For this review, take the finished solid that the model builds, in its own axes (mm). Face numbers are marked on the shaded views. A direction names the side the tool comes from. Coordinates: 2 decimals unless noted, no trailing zeros. Order: outer loops, then holes, each group sorted by start corner. A loop starts at its lowest first (then second) coordinate and runs counter-clockwise, first axis right, second up.
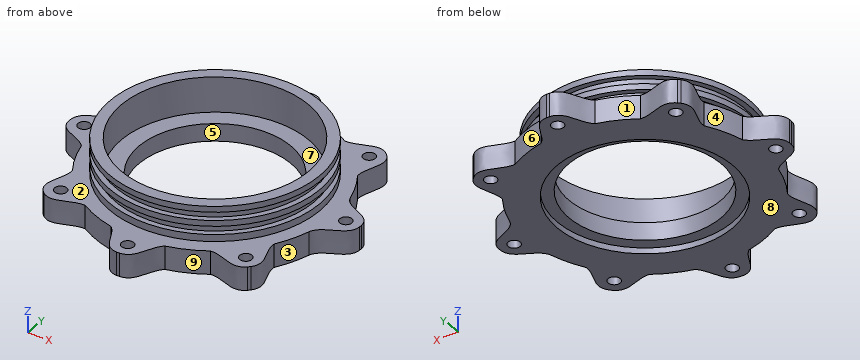
from build123d import *

# Parameters (mm, degrees)
SKETCH1_R           = 44.85
BOSS_EXTRUDE1_DEPTH = 15
SKETCH2_R           = 62.5
BOSS_EXTRUDE2_DEPTH = 10
SKETCH3_R           = 40
CUT_EXTRUDE1_DEPTH  = 15
SKETCH4_W           = 3.5
SKETCH4_H           = 3.724799257
SKETCH7_R           = 2.6
CUT_EXTRUDE4_DEPTH  = 92.855865354
CIRPATTERN1_COUNT   = 8
SKETCH9_R           = 37.5
CUT_EXTRUDE6_DEPTH  = 2.5
SKETCH10_R          = 32.5
CUT_EXTRUDE7_DEPTH  = 92.207181735
CUT_EXTRUDE12_DEPTH = 10


with BuildPart() as part:
    # Sketch1 → Boss-Extrude1 (new body)
    with BuildSketch(Plane.XY):
        Circle(SKETCH1_R)
    extrude(amount=BOSS_EXTRUDE1_DEPTH)

    # Sketch2 → Boss-Extrude2 (add)
    with BuildSketch(Plane(origin=(0, 0, 0), x_dir=(-1, 0, 0), z_dir=(0, 0, -1))):
        Circle(SKETCH2_R)
    extrude(amount=BOSS_EXTRUDE2_DEPTH)

    # Sketch3 → Cut-Extrude1 (cut)
    with BuildSketch(Plane.XY.offset(15)):
        Circle(SKETCH3_R)
    extrude(amount=-CUT_EXTRUDE1_DEPTH, mode=Mode.SUBTRACT)

    # Sketch4 → Cut-Revolve1 (revolve, cut)
    with BuildSketch(Plane(origin=(0, 0, 0), x_dir=(0, 0, -1), z_dir=(1, 0, 0))):
        with Locations((-4.75, 44.412399629)):
            Rectangle(SKETCH4_W, SKETCH4_H)
        with Locations((-10.75, 44.412399629)):
            Rectangle(SKETCH4_W, SKETCH4_H)
    revolve(axis=Axis((0, 0, -42.713110189), (0, 0, 1)), mode=Mode.SUBTRACT)

    # Sketch7 → Cut-Extrude4 (cut, through all)
    with BuildSketch(Plane(origin=(0, 0, -10), x_dir=(-1, 0, 0), z_dir=(0, 0, -1))):
        with Locations((56.25, 0)):
            Circle(SKETCH7_R)
    cut_extrude4 = extrude(amount=-CUT_EXTRUDE4_DEPTH, mode=Mode.SUBTRACT)

    # CirPattern1: Cut-Extrude4 ×8 about axis
    cirpattern1_axis = Axis((0, 0, 0), (0, 0, 1))
    for i in range(1, CIRPATTERN1_COUNT):
        add(cut_extrude4.rotate(cirpattern1_axis, i * 360 / CIRPATTERN1_COUNT), mode=Mode.SUBTRACT)

    # Sketch9 → Cut-Extrude6 (cut)
    with BuildSketch(Plane(origin=(0, 0, -10), x_dir=(-1, 0, 0), z_dir=(0, 0, -1))):
        Circle(SKETCH9_R)
    extrude(amount=-CUT_EXTRUDE6_DEPTH, mode=Mode.SUBTRACT)

    # Sketch10 → Cut-Extrude7 (cut, through all)
    with BuildSketch(Plane(origin=(0, 0, -7.5), x_dir=(-1, 0, 0), z_dir=(0, 0, -1))):
        Circle(SKETCH10_R)
    extrude(amount=-CUT_EXTRUDE7_DEPTH, mode=Mode.SUBTRACT)

    # Sketch16 → Cut-Extrude12 (cut)
    with BuildSketch(Plane.XY):
        with BuildLine():
            ThreePointArc((43.328890761, 26.899948428), (46.799594325, 20.268151644), (49.262217141, 13.1997713))
            add(Edge.make_bspline(
                [(62.49659969, 0.651941114), (62.158853916, 8.013585107), (51.562803867, 6.904158473), (49.262217141, 13.1997713)],
                knots=[0.027770853, 0.027770853, 0.027770853, 0.027770853, 1, 1, 1, 1], degree=3))
            ThreePointArc((62.49659969, 0.651941114), (57.723829207, 23.962669753), (44.584603378, 43.800264173))
            add(Edge.make_bspline(
                [(44.584603378, 43.800264173), (49.25969449, 38.753062003), (42.704327463, 32.585285285), (43.328890761, 26.899948428)],
                knots=[0.023286113, 0.023286113, 0.023286113, 0.023286113, 0.913122258, 0.913122258, 0.913122258, 0.913122258], degree=3))
        make_face()
        with BuildLine():
            add(Edge.make_bspline(
                [(62.49659969, -0.651941114), (62.158853916, -8.013585107), (51.562803867, -6.904158473), (49.262217141, -13.1997713)],
                knots=[0.027770853, 0.027770853, 0.027770853, 0.027770853, 1, 1, 1, 1], degree=3))
            ThreePointArc((49.262217141, -13.1997713), (46.799594325, -20.268151644), (43.328890761, -26.899948428))
            add(Edge.make_bspline(
                [(44.584603378, -43.800264173), (49.25969449, -38.753062003), (42.704327463, -32.585285285), (43.328890761, -26.899948428)],
                knots=[0.023286113, 0.023286113, 0.023286113, 0.023286113, 0.913122258, 0.913122258, 0.913122258, 0.913122258], degree=3))
            ThreePointArc((44.584603378, -43.800264173), (57.723829207, -23.962669753), (62.49659969, -0.651941114))
        make_face()
        with BuildLine():
            ThreePointArc((11.617016531, 49.659288425), (19.516855051, 47.117856158), (26.899948428, 43.328890761))
            add(Edge.make_bspline(
                [(43.800264173, 44.584603378), (38.753062003, 49.25969449), (32.585285285, 42.704327463), (26.899948428, 43.328890761)],
                knots=[0.023286113, 0.023286113, 0.023286113, 0.023286113, 0.913122258, 0.913122258, 0.913122258, 0.913122258], degree=3))
            ThreePointArc((43.800264173, 44.584603378), (23.917714523, 57.742470782), (0.55461157, 62.4975392))
            add(Edge.make_bspline(
                [(0.55461157, 62.4975392), (7.429311079, 62.234416947), (7.155243343, 53.237795727), (11.617016531, 49.659288425)],
                knots=[0.023286113, 0.023286113, 0.023286113, 0.023286113, 0.913122258, 0.913122258, 0.913122258, 0.913122258], degree=3))
        make_face()
        with BuildLine():
            add(Edge.make_bspline(
                [(43.800264173, -44.584603378), (38.753062003, -49.25969449), (32.585285285, -42.704327463), (26.899948428, -43.328890761)],
                knots=[0.023286113, 0.023286113, 0.023286113, 0.023286113, 0.913122258, 0.913122258, 0.913122258, 0.913122258], degree=3))
            ThreePointArc((26.899948428, -43.328890761), (19.516855051, -47.117856158), (11.617016531, -49.659288425))
            add(Edge.make_bspline(
                [(0.55461157, -62.4975392), (7.429311079, -62.234416947), (7.155243343, -53.237795727), (11.617016531, -49.659288425)],
                knots=[0.023286113, 0.023286113, 0.023286113, 0.023286113, 0.913122258, 0.913122258, 0.913122258, 0.913122258], degree=3))
            ThreePointArc((0.55461157, -62.4975392), (23.917714523, -57.742470782), (43.800264173, -44.584603378))
        make_face()
        with BuildLine():
            ThreePointArc((-26.899948428, 43.328890761), (-19.516855051, 47.117856158), (-11.617016531, 49.659288425))
            add(Edge.make_bspline(
                [(-0.55461157, 62.4975392), (-7.429311079, 62.234416947), (-7.155243343, 53.237795727), (-11.617016531, 49.659288425)],
                knots=[0.023286113, 0.023286113, 0.023286113, 0.023286113, 0.913122258, 0.913122258, 0.913122258, 0.913122258], degree=3))
            ThreePointArc((-0.55461157, 62.4975392), (-23.917714523, 57.742470782), (-43.800264173, 44.584603378))
            add(Edge.make_bspline(
                [(-43.800264173, 44.584603378), (-38.753062003, 49.25969449), (-32.585285285, 42.704327463), (-26.899948428, 43.328890761)],
                knots=[0.023286113, 0.023286113, 0.023286113, 0.023286113, 0.913122258, 0.913122258, 0.913122258, 0.913122258], degree=3))
        make_face()
        with BuildLine():
            add(Edge.make_bspline(
                [(-0.55461157, -62.4975392), (-7.429311079, -62.234416947), (-7.155243343, -53.237795727), (-11.617016531, -49.659288425)],
                knots=[0.023286113, 0.023286113, 0.023286113, 0.023286113, 0.913122258, 0.913122258, 0.913122258, 0.913122258], degree=3))
            ThreePointArc((-11.617016531, -49.659288425), (-19.516855051, -47.117856158), (-26.899948428, -43.328890761))
            add(Edge.make_bspline(
                [(-43.800264173, -44.584603378), (-38.753062003, -49.25969449), (-32.585285285, -42.704327463), (-26.899948428, -43.328890761)],
                knots=[0.023286113, 0.023286113, 0.023286113, 0.023286113, 0.913122258, 0.913122258, 0.913122258, 0.913122258], degree=3))
            ThreePointArc((-43.800264173, -44.584603378), (-23.917714523, -57.742470782), (-0.55461157, -62.4975392))
        make_face()
        with BuildLine():
            ThreePointArc((-49.659288425, 11.617016531), (-47.117856158, 19.516855051), (-43.328890761, 26.899948428))
            add(Edge.make_bspline(
                [(-44.584603378, 43.800264173), (-49.25969449, 38.753062003), (-42.704327463, 32.585285285), (-43.328890761, 26.899948428)],
                knots=[0.023286113, 0.023286113, 0.023286113, 0.023286113, 0.913122258, 0.913122258, 0.913122258, 0.913122258], degree=3))
            ThreePointArc((-44.584603378, 43.800264173), (-57.742470782, 23.917714523), (-62.4975392, 0.55461157))
            add(Edge.make_bspline(
                [(-62.4975392, 0.55461157), (-62.234416947, 7.429311079), (-53.237795727, 7.155243343), (-49.659288425, 11.617016531)],
                knots=[0.023286113, 0.023286113, 0.023286113, 0.023286113, 0.913122258, 0.913122258, 0.913122258, 0.913122258], degree=3))
        make_face()
        with BuildLine():
            add(Edge.make_bspline(
                [(-44.584603378, -43.800264173), (-49.25969449, -38.753062003), (-42.704327463, -32.585285285), (-43.328890761, -26.899948428)],
                knots=[0.023286113, 0.023286113, 0.023286113, 0.023286113, 0.913122258, 0.913122258, 0.913122258, 0.913122258], degree=3))
            ThreePointArc((-43.328890761, -26.899948428), (-47.117856158, -19.516855051), (-49.659288425, -11.617016531))
            add(Edge.make_bspline(
                [(-62.4975392, -0.55461157), (-62.234416947, -7.429311079), (-53.237795727, -7.155243343), (-49.659288425, -11.617016531)],
                knots=[0.023286113, 0.023286113, 0.023286113, 0.023286113, 0.913122258, 0.913122258, 0.913122258, 0.913122258], degree=3))
            ThreePointArc((-62.4975392, -0.55461157), (-57.742470782, -23.917714523), (-44.584603378, -43.800264173))
        make_face()
    extrude(amount=-CUT_EXTRUDE12_DEPTH, mode=Mode.SUBTRACT)


solid = part.part
1. Machinability: for the marked faces 5, 6, 7, 8 and 9, which of the approach directions +Z, -Z, +X, -X, +Y, -Y give a long, thin tool a straight path to every point of the face, cutting with its end or side? Answer none if there is none.
Answer below:
face 5: +Z, -Z
face 6: +Z, -Z, +Y
face 7: +Z
face 8: -Z, +X, -X, +Y, -Y
face 9: +Z, -Z, -Y
2. To check wall thickness, follow L1, parallel to Z at x = 41, y = -45; L2, parallel to X at y = 36.5, z = 6; L3, parallel to X at y = 56.25, z = -6. State the ranges of each line that lie inside material, in increasing order.
Answer below:
L1: z = -10 to 0
L2: x = -21.87 to -16.36, 16.36 to 21.87
L3: x = -7.5 to -2.6, 2.6 to 7.5
3. Take a section at B-B, the plane z = -4.75. Give the number of separate pieces and of enclosed holes in the cut face, plus the area to 3 significant figures.
Answer below:
separate pieces: 1
enclosed holes: 9
area: 6,040 mm2
4. Take a section at A-A, the plane z = 10.75. Give the boundary of the cut face in (x, y), plus the area to 3 significant figures.
Answer below:
outline: circle Ø85.1 at (0, 0); hole circle Ø80 at (0, 0)
area: 661 mm2
5. The part is to be moulded in two halves that separate along X. For the marked faces 1, 2, 3 and 4, say which applies: +X half, -X half, draft (parallel to the pull), parting line (faces both ways), or undercut.
Answer below:
face 1: undercut
face 2: draft
face 3: +X half
face 4: -X half
6. Clearance check with flat-ended pins moving along their axes: pin 1 Ø1 at (y, z) = (6, 0) entering from +X; pin 2 Ø3 at (x, z) = (-11, -5.5) entering from -Y; pin 3 Ø1.5 at (x, z) = (6, -5.5) entering from +Y. State where each tip first meets the part, or that it passes through.
Answer below:
pin 1: stops at x = 59.82
pin 2: stops at y = -52.2
pin 3: stops at y = 60.15
